from build123d import *

# Parameters (mm, degrees)
BOSS_EXTRUDE1_DEPTH   = 25
BOSS_EXTRUDE1_2_DEPTH = 25
BOSS_EXTRUDE1_3_DEPTH = 25
BOSS_EXTRUDE1_4_DEPTH = 25
BOSS_EXTRUDE1_5_DEPTH = 25
BOSS_EXTRUDE1_6_DEPTH = 25
BOSS_EXTRUDE2_DEPTH   = 15
SKETCH3_R             = 1.5499999999999976
SKETCH3_R_2           = 1.5499999999999996
SKETCH3_R_3           = 1.5499999999999958
SKETCH3_W             = 5.4
SKETCH3_H             = 2
SKETCH3_W_2           = 2
SKETCH3_H_2           = 5.400000000000006
CUT_EXTRUDE1_DEPTH    = 51.449536703397406
SKETCH4_R             = 4.000000000000001
SKETCH4_R_2           = 4
SKETCH4_R_3           = 3.9999999999999973
CUT_EXTRUDE2_DEPTH    = 10
CUT_EXTRUDE12_DEPTH   = 9
SKETCH18_R            = 7.5
CUT_EXTRUDE13_DEPTH   = 3
FILLET1_R             = 10


with BuildPart() as part:
    # Sketch1 → Boss-Extrude1 (new body)
    with BuildSketch(Plane(origin=(0, 0, 0), x_dir=(1, 0, 0), z_dir=(0, 1, 0))):
        Polygon((-3.4999999999999987, -4.3500000000000005), (-9.208219674195641, -4.350000000000002), (-12.827870678242386, -2.260193518441092), (-9.011473670974864, 4.35), (-3.499999999999964, 4.35), (-3.4999999999999636, 1.35), (-6.499999999999999, 1.3499999999999996), (-6.499999999999999, -1.3500000000000005), (-3.4999999999999987, -1.3500000000000008), align=None)
    extrude(amount=BOSS_EXTRUDE1_DEPTH)



with BuildPart() as body_2:
    # Sketch1 → Boss-Extrude1 2 (new body)
    with BuildSketch(Plane(origin=(0, 0, 0), x_dir=(1, 0, 0), z_dir=(0, 1, 0))):
        Polygon((-21.327870678242448, -16.982625382776504), (-16.414613987909505, -19.81929545553799), (-10.481908744213749, -19.819295455538416), (-10.48190874421371, -16.31634119473297), (-13.391525876671139, -14.636472960069911), (-14.891525876671151, -17.23454917142322), (-16.06066017178014, -16.559549171423214), (-17.22979446688913, -15.884549171423206), (-15.729794466888796, -13.286472960069348), (-18.327870678242103, -11.786472960069336), align=None)
    extrude(amount=BOSS_EXTRUDE1_2_DEPTH)


with BuildPart() as body_3:
    # Sketch1 → Boss-Extrude1 3 (new body)
    with BuildSketch(Plane(origin=(0, 0, 0), x_dir=(1, 0, 0), z_dir=(0, 1, 0))):
        Polygon((9.011473670974846, 4.350000000000008), (7.500000000000001, 4.35), (7.500000000000003, -4.35), (12.400815759693463, -1.5205127018921853), align=None)
    extrude(amount=BOSS_EXTRUDE1_3_DEPTH)


with BuildPart() as body_4:
    # Sketch1 → Boss-Extrude1 4 (new body)
    with BuildSketch(Plane(origin=(0, 0, 0), x_dir=(1, 0, 0), z_dir=(0, 1, 0))):
        Polygon((21.3278706782425, -16.982625382776575), (16.4146139879095, -19.819295455537993), (10.481908744213753, -19.819295455538413), (10.481908744213746, -16.316341194733052), (13.391525876671182, -14.636472960069986), (14.891525876671192, -17.234549171423296), (16.060660171780043, -16.559549171423036), (17.22979446688917, -15.884549171423286), (15.729794466888857, -13.286472960069448), (18.32787067824215, -11.78647296006941), align=None)
    extrude(amount=BOSS_EXTRUDE1_4_DEPTH)


with BuildPart() as body_5:
    # Sketch1 → Boss-Extrude1 5 (new body)
    with BuildSketch(Plane(origin=(0, 0, 0), x_dir=(1, 0, 0), z_dir=(0, 1, 0))):
        Polygon((9.999999999999996, -35.27894572633552), (11.349999999999998, -35.27894572633552), (11.349999999999998, -32.27894572633372), (14.349999999999998, -32.27894572633372), (14.349999999999998, -38.27894572633372), (5.649999999999999, -38.27894572633372), (5.649999999999998, -32.27894572633428), (8.649999999999999, -32.27894572633428), (8.649999999999999, -35.27894572633552), align=None)
    extrude(amount=BOSS_EXTRUDE1_5_DEPTH)


with BuildPart() as body_6:
    # Sketch1 → Boss-Extrude1 6 (new body)
    with BuildSketch(Plane(origin=(0, 0, 0), x_dir=(1, 0, 0), z_dir=(0, 1, 0))):
        Polygon((-5.649999999999998, -32.27894572633428), (-5.649999999999999, -38.27894572633372), (-14.349999999999998, -38.27894572633372), (-14.349999999999998, -32.27894572633372), (-11.349999999999998, -32.27894572633372), (-11.349999999999998, -35.27894572633552), (-9.999999999999996, -35.27894572633552), (-8.649999999999999, -35.27894572633552), (-8.649999999999999, -32.27894572633428), align=None)
    extrude(amount=BOSS_EXTRUDE1_6_DEPTH)


with BuildPart() as part_1:
    add(part.part)

    add(body_2.part)  # Boss-Extrude2 merges body 2

    add(body_3.part)  # Boss-Extrude2 merges body 3

    add(body_4.part)  # Boss-Extrude2 merges body 4

    add(body_5.part)  # Boss-Extrude2 merges body 5

    add(body_6.part)  # Boss-Extrude2 merges body 6
    # Sketch2 → Boss-Extrude2 (add)
    with BuildSketch(Plane(origin=(0, 0, 0), x_dir=(-1, 0, 0), z_dir=(0, -1, 0))):
        Polygon((-21.3278706782425, -16.982625382776575), (-9.011473670974844, 4.350000000000008), (9.011473670974864, 4.35), (21.327870678242448, -16.982625382776515), (21.327870678242448, -38.27894572633375), (-21.3278706782425, -38.27894572633371), align=None)
    extrude(amount=BOSS_EXTRUDE2_DEPTH)

    # Sketch3 → Cut-Extrude1 (cut, through all)
    with BuildSketch(Plane(origin=(0, 0, 0), x_dir=(1, 0, 0), z_dir=(0, 1, 0))):
        with Locations(Location((-15.327870678242446, -24.278945726333717, 0), (0, 0, 270))):
            Circle(SKETCH3_R)
        with Locations(Location((1.55e-15, -6.649999999999997, 0), (0, 0, 270))):
            Circle(SKETCH3_R_2)
        with Locations(Location((15.327870678242453, -24.278945726333713, 0), (0, 0, 90))):
            Circle(SKETCH3_R_3)
        with Locations((0.10000000000000098, 0)):
            Rectangle(SKETCH3_W, SKETCH3_H)
        Polygon((-14.976685575564561, -12.682050096663907), (-13.244634767995688, -13.682050096663914), (-10.54463476799567, -9.005512916227953), (-12.276685575564542, -8.005512916227948), align=None)
        Polygon((11.000000000000004, -25.978945726335514), (9.000000000000004, -25.978945726335514), (9.000000000000007, -31.37894572633552), (11.000000000000007, -31.37894572633552), align=None)
        with Locations((-9.999999999999996, -28.678945726335517)):
            Rectangle(SKETCH3_W_2, SKETCH3_H_2)
        Polygon((10.544634767995705, -9.005512916227941), (12.27668557556458, -8.005512916227937), (14.976685575564584, -12.682050096663904), (13.244634767995707, -13.682050096663906), align=None)
    extrude(amount=-CUT_EXTRUDE1_DEPTH, mode=Mode.SUBTRACT)

    # Sketch4 → Cut-Extrude2 (cut)
    with BuildSketch(Plane(origin=(0, 0, 0), x_dir=(1, 0, 0), z_dir=(0, 1, 0))):
        with Locations(Location((-15.327870678242446, -24.278945726333717, 0), (0, 0, 270))):
            Circle(SKETCH4_R)
        with Locations(Location((1.55e-15, -6.649999999999996, 0), (0, 0, 270))):
            Circle(SKETCH4_R_2)
        with Locations(Location((15.327870678242453, -24.278945726333713, 0), (0, 0, 270))):
            Circle(SKETCH4_R_3)
    extrude(amount=-CUT_EXTRUDE2_DEPTH, mode=Mode.SUBTRACT)

    # Sketch17 → Cut-Extrude12 (cut)
    with BuildSketch(Plane(origin=(0, -15, 0), x_dir=(-1, 0, 0), z_dir=(0, -1, 0))):
        Polygon((7.011473670974844, -3.6499999999999915), (-7.011473670974842, -3.6499999999999932), (-21.32787067824244, -21.982625382776526), (-21.32787067824244, -16.982625382776508), (-9.011473670974846, 4.350000000000003), (9.011473670974864, 4.35), (21.327870678242448, -16.982625382776515), (21.327870678242448, -21.98262538277652), align=None)
    extrude(amount=-CUT_EXTRUDE12_DEPTH, mode=Mode.SUBTRACT)

    # Sketch18 → Cut-Extrude13 (cut)
    with BuildSketch(Plane(origin=(0, -15, 0), x_dir=(-1, 0, 0), z_dir=(0, -1, 0))):
        with Locations(Location((0, -17.650000000000002, 0), (0, 0, 90))):
            Circle(SKETCH18_R)
    extrude(amount=-CUT_EXTRUDE13_DEPTH, mode=Mode.SUBTRACT)

    # Fillet1
    fillet1_edges = [part_1.edges().sort_by_distance(p)[0] for p in [
        (-9.011473670974864, 9.5, -4.35),
        (9.011473670974846, 9.5, -4.350000000000008),
    ]]
    fillet(fillet1_edges, radius=FILLET1_R)


solid = part_1.part
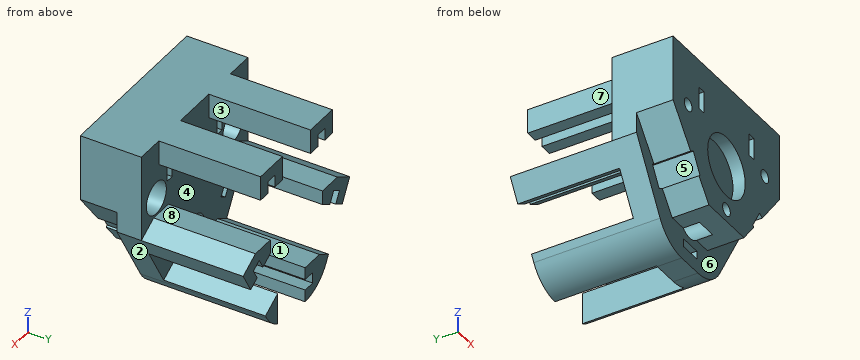
CAD build for the part. Positions are in the model's coordinates, mm. Face numbers are marked on the shaded views. A direction names the side the tool comes from. Give positions to 0.01 mm unless a question says otherwise; leave off trailing zeros. Order: outer loops, then holes, each group sorted by start corner. A loop starts at its lowest first (then second) coordinate and runs counter-clockwise, first axis right, second up. Notation, with made-up numbers: (74, 1.5) - (98, 1.5) arc R32 cw to (98, 34.5) - close; hole circle Ø9 at (48, 61.25). An arc over 180 degrees is marked (long way). Answer in a Markdown table with one row per item.
1. Saw through at D-D, the plane z = 6.65. Give the cut face in (x, y).
Data:
| item | result |
|---|---|
| outline | (-15.36, -6) - (-9.35, -6) - (-9.35, -15) - (-1.55, -15) - (-1.55, -10) - (-4, -10) - (-4, 0) - (-15.36, 0) - close; (1.55, -15) - (9.35, -15) - (9.35, -6) - (15.36, -6) - (15.36, 0) - (4, 0) - (4, -10) - (1.55, -10) - close |
2. Saw through at C-C, the plane y = 13. Count the separate pieces of the cut face and the enclosed holes in it, plus the area to 3 significant figures.
Data:
| item | result |
|---|---|
| separate pieces | 6 |
| enclosed holes | 0 |
| area | 254 mm² |
3. Pull direction Z, two halves, no side cores. Call the marked faces 1, 2, 3 and 4: pulls with the +Z half, pulls with the -Z half, needs draft (parallel to the pull), parting line crosses it, or undercut.
Data:
| item | result |
|---|---|
| face 1 | undercut |
| face 2 | pulls with the -Z half |
| face 3 | needs draft |
| face 4 | undercut |
4. Saw through at B-B, the plane x = 0. Give the cut face in (y, z), plus the area to 3 significant figures.
Data:
| item | result |
|---|---|
| outline | (-15, 3.65) - (-10, 3.65) - (-10, 5.1) - (-15, 5.1) - close; (-15, 8.2) - (-10, 8.2) - (-10, 10.65) - (0, 10.65) - (0, 38.28) - (-15, 38.28) - (-15, 25.15) - (-12, 25.15) - (-12, 10.15) - (-15, 10.15) - close; (-6, -4.35) - (0, -4.35) - (0, -1) - (-6, -1) - close; (-6, 1) - (0, 1) - (0, 2.65) - (-6, 2.65) - close |
| area | 419 mm² |
5. Tool access for the marked faces 5, 6, 7 and 8: list every direction of +Z, -Z, +X, -X, +Y, -Y with a clear straight run to the whole face (end or side of a thin tool).
Data:
| item | result |
|---|---|
| face 5 | +Y, -Y |
| face 6 | -Z, -Y |
| face 7 | +Z, -X, +Y |
| face 8 | +X, -X, +Y |
6. Flat gauge pins, fed straight in: pin 1 (3.5 mm diameter, centred on x = 7.5, y = 16.5, fed in from -Z); pin 2 (3 mm diameter, centred on x = 5.5, y = 20.5, fed in from -Z); pin 3 (2 mm diameter, centred on x = -13, y = 2, fed in from -Z). Where does each tip first touch, or does it go through?
Data:
| item | result |
|---|---|
| pin 1 | stops at z = -3.4 |
| pin 2 | stops at z = 32.28 |
| pin 3 | stops at z = 0.83 |
7. Probe probe 1 along X at (y, z) = (23, 33); probe 2 along Z at (x, y) = (-11.5, 19); probe 3 along Y at (x, z) = (-6.5, 27). List the from-to ranges inside material, lowest first. Write a range as [from, to].
Data:
| item | result |
|---|---|
| probe 1 | x = [-14.35, -11.35], [-8.65, -5.65], [5.65, 8.65], [11.35, 14.35] |
| probe 2 | z = [0.02, 3.03], [15.73, 19.82], [32.28, 38.28] |
| probe 3 | y = [-15, 0] |
8. Saw through at A-A, the plane z = 29. Give the cut face in (x, y).
Data:
| item | result |
|---|---|
| outline | (-21.33, -15) - (-11, -15) - (-11, 0) - (-21.33, 0) - close; (-9, -15) - (9, -15) - (9, 0) - (-9, 0) - close; (11, -15) - (21.33, -15) - (21.33, 0) - (11, 0) - close |
